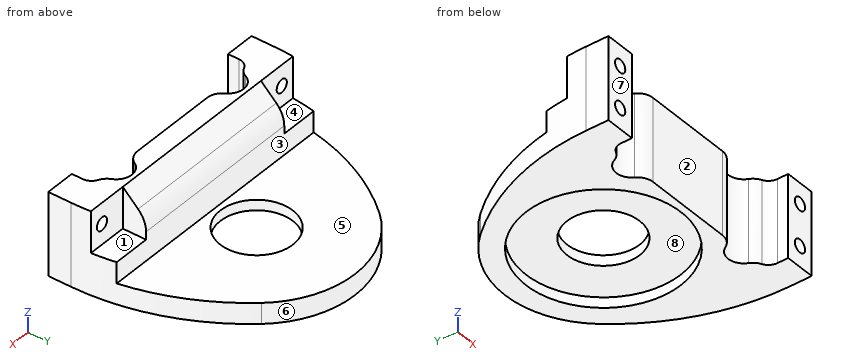
```python
from build123d import *

# Parameters (mm, degrees)
ESBO_O1_R                     = 14.95
RESSALTO_EXTRUS_O1_DEPTH      = 2
ESBO_O2_R                     = 7
RESSALTO_EXTRUS_O2_DEPTH      = 2
ESBO_O3_W                     = 49.96
ESBO_O3_H                     = 12
RESSALTO_EXTRUS_O3_DEPTH      = 8.1
CHANFRO1_SIZE                 = 12.5
CHANFRO1_SIZE_2               = 12
FILETE1_R                     = 44
CORTE_EXTRUS_O1_REACH         = 38.116
CORTE_EXTRUS_O2_DEPTH         = 37.115930003
ESBO_O7_W                     = 49.64413541
ESBO_O7_H                     = 12
CORTE_EXTRUS_O5_DEPTH         = 8
FILETE2_R                     = 5
FURO_ROSCADO_DE_M3X0_51_D     = 2.5
FURO_ROSCADO_DE_M3X0_51_DEPTH = 8.5
FURO_ROSCADO_DE_M3X0_51_TIP   = 0.751075774
CORTE_EXTRUS_O6_DEPTH         = 8
FILETE3_R                     = 3


with BuildPart() as part:
    # Esboço1 → Ressalto-extrusão1 (new body)
    with BuildSketch(Plane.XY):
        with BuildLine():
            Line((-24.98, -20.6), (-24.98, 0))
            Line((-24.98, 0), (-14.451561249, 12.33500618))
            ThreePointArc((-14.451561249, 12.33500618), (0, 19), (14.451561249, 12.33500618))
            Line((14.451561249, 12.33500618), (24.98, 0))
            Line((24.98, 0), (24.98, -20.6))
            Line((24.98, -20.6), (18.98, -20.6))
            Line((18.98, -20.6), (-18.98, -20.6))
            Line((-18.98, -20.6), (-24.98, -20.6))
        make_face()
        Circle(ESBO_O1_R, mode=Mode.SUBTRACT)
    extrude(amount=RESSALTO_EXTRUS_O1_DEPTH)

    # Esboço2 → Ressalto-extrusão2 (add)
    with BuildSketch(Plane.XY.offset(2)):
        with BuildLine():
            Line((24.98, 0), (14.451561249, 12.33500618))
            ThreePointArc((14.451561249, 12.33500618), (0, 19), (-14.451561249, 12.33500618))
            Line((-14.451561249, 12.33500618), (-24.98, 0))
            Line((-24.98, 0), (-24.98, -20.6))
            Line((-24.98, -20.6), (24.98, -20.6))
            Line((24.98, -20.6), (24.98, 0))
        make_face()
        Circle(ESBO_O2_R, mode=Mode.SUBTRACT)
    extrude(amount=RESSALTO_EXTRUS_O2_DEPTH)

    # Esboço3 → Ressalto-extrusão3 (add)
    with BuildSketch(Plane.XZ.offset(20.6)):
        with Locations((0, 10)):
            Rectangle(ESBO_O3_W, ESBO_O3_H)
    extrude(amount=-RESSALTO_EXTRUS_O3_DEPTH)

    # Chanfro1
    # the kernel refuses this chamfer: 12.5, 12 mm, written as the material it adds along each edge
    with BuildSketch(Plane(origin=(-24.98, -12.5, 4), x_dir=(-1.156063365908983e-15, 0.9996377364334812, -0.026914603808079415), z_dir=(1, 0, 0))) as chanfro1_piece_1_section:
        Polygon((CHANFRO1_SIZE * 0.999637736433, CHANFRO1_SIZE * 0.0269146038081), (-CHANFRO1_SIZE_2 * 0.0269146038081, CHANFRO1_SIZE_2 * 0.999637736433), (0, 0), align=None)
    chanfro1_piece_1 = extrude(amount=49.96, mode=Mode.PRIVATE)
    chanfro1_piece_1 = chanfro1_piece_1 - Plane(origin=(0, 0, 8.125756992), x_dir=(1, 0, 0), z_dir=(0, 0, -1)) * Cylinder(7, 150, mode=Mode.PRIVATE)
    add(chanfro1_piece_1)

    # Filete1
    # the kernel refuses this fillet: 44 mm, written as the material it takes off along each edge
    with BuildSketch(Plane(origin=(-24.98, 0, 44.561650607), x_dir=(0.6492108903913877, 0.7606084536719413, 0), z_dir=(0, 0, -1)), Plane(origin=(24.98, 0, -40.561650607), x_dir=(-0.6492108903913875, 0.7606084536719414, 0), z_dir=(0, 0, 1))) as filete1_piece_1:
        with BuildLine():
            CenterArc((16.224665438, 43.999998084), FILETE1_R, 229.517867219, 40.465225033)
            Line((-12.340613739, 10.533226123), (-15.197141656, 7.186548926))
            Line((-15.197141656, 7.186548926), (-1.622466416, -4.399999917))
            Line((-1.622466416, -4.399999917), (16.210382799, -4.399999808))
            Line((16.210382799, -4.399999808), (16.211681221, 0))
        make_face()
    extrude(amount=85.123301215, mode=Mode.SUBTRACT)

    # Esboço4 → Corte-extrusão1 (cut, up to next)
    with BuildSketch(Plane.XY.offset(16), mode=Mode.PRIVATE) as corte_extrus_o1_sk1:
        with BuildLine():
            Line((17, -16.5), (-17, -16.5))
            ThreePointArc((-17, -16.5), (-18.414213562, -17.085786438), (-19, -18.5))
            Line((-19, -18.5), (-19, -20.6))
            Line((-19, -20.6), (19, -20.6))
            Line((19, -20.6), (19, -18.5))
            ThreePointArc((19, -18.5), (18.414213562, -17.085786438), (17, -16.5))
        make_face()
    corte_extrus_o1_tool1 = extrude(corte_extrus_o1_sk1.sketch, amount=-CORTE_EXTRUS_O1_REACH, mode=Mode.PRIVATE) & part.part
    add(corte_extrus_o1_tool1.solids().sort_by_distance((0, -18.567864, 16))[0], mode=Mode.SUBTRACT)

    # Esboço6 → Corte-extrusão2 (cut, through all)
    with BuildSketch(Plane(origin=(0, 0, 0), x_dir=(-1, 0, 0), z_dir=(0, 0, -1))):
        with BuildLine():
            Line((17, -16.3), (16.75, -16.3))
            ThreePointArc((16.75, -16.3), (14.526457135, -13.402222521), (11.151923789, -14.8))
            ThreePointArc((11.151923789, -14.8), (10.053847577, -15.898076211), (8.553847577, -16.3))
            Line((8.553847577, -16.3), (-8.553847577, -16.3))
            ThreePointArc((-8.553847577, -16.3), (-10.053847577, -15.898076211), (-11.151923789, -14.8))
            ThreePointArc((-11.151923789, -14.8), (-14.526457135, -13.402222521), (-16.75, -16.3))
            Line((-16.75, -16.3), (-17, -16.3))
            ThreePointArc((-17, -16.3), (-18.555634919, -16.944365081), (-19.2, -18.5))
            Line((-19.2, -18.5), (-19.2, -20.6))
            Line((-19.2, -20.6), (19.2, -20.6))
            Line((19.2, -20.6), (19.2, -18.5))
            ThreePointArc((19.2, -18.5), (18.555634919, -16.944365081), (17, -16.3))
        make_face()
    extrude(amount=-CORTE_EXTRUS_O2_DEPTH, mode=Mode.SUBTRACT)

    # Esboço7 → Corte-extrusão5 (cut)
    with BuildSketch(Plane(origin=(0, 0, 0), x_dir=(-1, 0, 0), z_dir=(0, -1, 0))):
        with Locations((0, -10)):
            Rectangle(ESBO_O7_W, ESBO_O7_H)
    extrude(amount=CORTE_EXTRUS_O5_DEPTH, mode=Mode.SUBTRACT)

    # Filete2
    filete2_edges = [part.edges().sort_by_distance(p)[0] for p in [
        (0, -8, 11.68),
    ]]
    fillet(filete2_edges, radius=FILETE2_R)

    # Furo roscado de M3x0.51
    with Locations(Plane.XZ.offset(20.6)):
        with Locations((22.09, 4), (22.09, 12), (-22.09, 4), (-22.09, 12)):
            Hole(FURO_ROSCADO_DE_M3X0_51_D / 2, depth=FURO_ROSCADO_DE_M3X0_51_DEPTH)
            with Locations((0, 0, -(FURO_ROSCADO_DE_M3X0_51_DEPTH + FURO_ROSCADO_DE_M3X0_51_TIP / 2))):  # 118° drill point
                Cone(0, FURO_ROSCADO_DE_M3X0_51_D / 2, FURO_ROSCADO_DE_M3X0_51_TIP, mode=Mode.SUBTRACT)

    # Esboço12 → Corte-extrusão6 (cut)
    with BuildSketch(Plane(origin=(24.98, 0, 0), x_dir=(0, 0, -1), z_dir=(1, 0, 0))):
        with BuildLine():
            Line((-9.54891062, -12.5), (-8.04891062, -12.5))
            Line((-8.04891062, -12.5), (-8.04891062, -8))
            Line((-8.04891062, -8), (-9.54891062, -8))
            ThreePointArc((-9.54891062, -8), (-11.509357545, -8.400364378), (-13.155847225, -9.537340859))
            Line((-13.155847225, -9.537340859), (-16, -12.5))
            Line((-16, -12.5), (-9.54891062, -12.5))
        make_face()
    corte_extrus_o6 = extrude(amount=-CORTE_EXTRUS_O6_DEPTH, mode=Mode.SUBTRACT)

    # Espelhar1: Corte-extrusão6 across plane
    add(corte_extrus_o6.mirror(Plane(origin=(0, 0, 0), x_dir=(0, 0, 1), z_dir=(1, 0, 0))), mode=Mode.SUBTRACT)

    # Filete3
    filete3_edges = [part.edges().sort_by_distance(p)[0] for p in [
        (16.75, -16.3, 8),
        (-16.75, -16.3, 8),
    ]]
    fillet(filete3_edges, radius=FILETE3_R)


solid = part.part
```
Geometry: final body of the model. Coordinates: model frame, mm. Face numbers are marked on the shaded views. A direction names the side the tool comes from. Coordinates: 2 decimals unless noted, no trailing zeros. Order: outer loops, then holes, each group sorted by start corner. A loop starts at its lowest first (then second) coordinate and runs counter-clockwise, first axis right, second up. Notation, with made-up numbers: (62.5, 54.25) - (89.5, 54.25) arc R32 cw to (89.5, 83.25) - close; hole circle Ø6 at (53.5, 33.25). An arc over 180 degrees is marked (long way). Return JSON: item names as keys, results as strings. Group by question number.
1. Pull-direction query (Y, two-part tool) for the marked faces 5, 6, 7 and 8; classes: pulls with the +Y half, pulls with the -Y half, needs draft (parallel to the pull), parting line crosses it, or undercut.
2. Cut plane D-D (z = 12). Count the separate pieces of the cut face and the enclosed holes in it, plus the area to 3 significant figures.
3. Material intervals for line 1 along Z through (x, y) = (22.09, -18.75); line 2 along X through (y, z) = (-15, 4.5); line 3 along X through (y, z) = (-16, 3.5), sorted ascending. Write a range as [from, to].
4. Pin query (flat end, axial travel): pin 1 (21.5 mm diameter, centred on x = -7, y = 8.5, fed in from +Z); pin 2 (2.5 mm diameter, centred on x = -20.5, y = -11, fed in from +Z); pin 3 (3 mm diameter, centred on x = -7, y = -3.5, fed in from -Z). Return the tip coordinate at first contact, or that it passes through.
5. Cut plane B-B (y = 4.5). Output: boundary loops of the cut face in (x, z), plus the area to 3 significant figures.
6. Set-up query: the marked faces 1, 2, 3 and 4. Return all of +Z, -Z, +X, -X, +Y, -Y with unobstructed straight access to the full face (end or side cutting, diameter ignored); none if empty.
7. Cut plane C-C (x = 10). Output: boundary loops of the cut face in (y, z), plus the area to 3 significant figures.
8. Cut plane A-A (x = 0). Output: boundary loops of the cut face in (y, z).
Resolved:
{
 "1": {"face 5": "needs draft", "face 6": "pulls with the +Y half", "face 7": "pulls with the -Y half", "face 8": "undercut"},
 "2": {"separate pieces": "3", "enclosed holes": "0", "area": "301 mm²"},
 "3": {"line 1": "z = [0, 2.75], [5.25, 10.75], [13.25, 16]", "line 2": "x = [-24.96, -23.24], [-20.94, -16.45], [-11.03, 11.03], [16.45, 20.94], [23.24, 24.96]", "line 3": "x = [-24.98, -23.24], [-20.94, -17.17], [-9.86, 9.86], [17.17, 20.94], [23.24, 24.98]"},
 "4": {"pin 1": "stops at z = 4", "pin 2": "stops at z = 8.05", "pin 3": "stops at z = 2"},
 "5": {"outline": "(-19.79, 0) - (-14.26, 0) - (-14.26, 2) - (-5.36, 2) - (-5.36, 4) - (-19.79, 4) - close; (5.36, 2) - (14.26, 2) - (14.26, 0) - (19.79, 0) - (19.79, 4) - (5.36, 4) - close", "area": "79.9 mm²"},
 "6": {"face 1": "+Z, +X, +Y", "face 2": "+Z, -Z, -Y", "face 3": "+Z, +X, -X, +Y", "face 4": "+Z, -X, +Y"},
 "7": {"outline": "(-15.93, 0) - (-11.11, 0) - (-11.11, 2) - (11.11, 2) - (11.11, 0) - (16.16, 0) - (16.16, 4) - (-8, 4) - (-8, 9.55) arc R5 ccw to (-9.54, 13.16) - (-12.5, 16) - (-15.93, 16) - close", "area": "169 mm²"},
 "8": {"outline": "(-16.3, 0) - (-14.95, 0) - (-14.95, 2) - (-7, 2) - (-7, 4) - (-8, 4) - (-8, 9.55) arc R5 ccw to (-9.54, 13.16) - (-12.5, 16) - (-16.3, 16) - close; (7, 2) - (14.95, 2) - (14.95, 0) - (19, 0) - (19, 4) - (7, 4) - close"}
}
